```python
from build123d import *

# Parameters (mm, degrees)
F2_DEPTH  = 304.8
F4_D      = 14.2875
F4_DEPTH  = 6.35
F6_D      = 38.1
F6_DEPTH  = 6.35
F8_D      = 14.2875
F8_DEPTH  = 6.35
F10_D     = 31.75
F10_DEPTH = 6.35


with BuildPart() as f2:
    # F1 (on Right) → F2 (new body, symmetric)
    with BuildSketch(Plane.YZ):
        with BuildLine():
            Line((-177.776466, 50.8), (-266.676466, 50.8))
            ThreePointArc((-266.676466, 50.8), (-271.166595, 48.940128), (-273.026466, 44.45))
            Line((-273.026466, 44.45), (-273.026466, 37.770297))
            Line((-273.026466, 37.770297), (-273.026466, 6.35))
            ThreePointArc((-273.026466, 6.35), (-271.166595, 1.859872), (-266.676466, 0))
            Line((-266.676466, 0), (-177.776466, 0))
            ThreePointArc((-177.776466, 0), (-173.286338, 1.859872), (-171.426466, 6.35))
            Line((-171.426466, 6.35), (-171.426466, 44.45))
            ThreePointArc((-171.426466, 44.45), (-173.286338, 48.940128), (-177.776466, 50.8))
        make_face()
        with BuildLine():
            ThreePointArc((-266.671124, 38.101069), (-264.810874, 42.590506), (-260.321124, 44.45))
            Line((-260.321124, 44.45), (-182.185624, 44.45))
            ThreePointArc((-182.185624, 44.45), (-177.695496, 42.590128), (-175.835624, 38.1))
            Line((-175.835624, 38.1), (-175.835624, 12.7))
            ThreePointArc((-175.835624, 12.7), (-177.695496, 8.209872), (-182.185624, 6.35))
            Line((-182.185624, 6.35), (-260.325398, 6.35))
            ThreePointArc((-260.325398, 6.35), (-264.815904, 8.21025), (-266.675398, 12.701069))
            Line((-266.675398, 12.701069), (-266.671124, 38.101069))
        make_face(mode=Mode.SUBTRACT)
    extrude(amount=F2_DEPTH, both=True)

    # F4
    with Locations(Plane.XY.offset(50.8)):
        with Locations((-85.725, -222.226466), (85.725, -222.226466)):
            Hole(F4_D / 2, depth=F4_DEPTH)

    # F6
    with Locations(Plane.XY.offset(50.8)):
        with Locations((-228.6, -222.226466)):
            Hole(F6_D / 2, depth=F6_DEPTH)

    # F8
    with Locations(Plane(origin=(0, 0, 0), x_dir=(1, 0, 0), z_dir=(0, 0, -1))):
        with Locations((-228.6, 222.226466)):
            Hole(F8_D / 2, depth=F8_DEPTH)

    # F10
    with Locations(Plane(origin=(0, 0, 0), x_dir=(1, 0, 0), z_dir=(0, 0, -1))):
        with Locations((-85.725, 222.226466), (85.725, 222.226466)):
            Hole(F10_D / 2, depth=F10_DEPTH)


solid = f2.part
```
Input: part model. Units: mm. Frame: model coordinates. A direction names the side the tool comes from. Round coordinates to 2 decimals unless told otherwise and drop trailing zeros. Loops run counter-clockwise (first coordinate to the right, second up) from the corner with the lowest first, then second, coordinate; pieces in that order, holes last. Notation, with made-up numbers: (-28, 44.25) -> (-21, 44.25) arc R22 ccw to (-21, 66.25) -> close; hole circle Ø10 at (27.25, 48). An arc over 180 degrees is marked (long way). One line per item, written item: value.
(1) Section B-B (z = 19.5). Return the cut outline in (x, y), plus the area to 3 significant figures.
Geometry check:
outline: (-304.8, -273.03) -> (304.8, -273.03) -> (304.8, -266.67) -> (-304.8, -266.67) -> close; (-304.8, -175.84) -> (304.8, -175.84) -> (304.8, -171.43) -> (-304.8, -171.43) -> close
area: 6,560 mm2
(2) Material intervals for line 1 (Z direction, x = -90, y = -250.5); line 2 (Z direction, x = -235.5, y = -261); line 3 (Y direction, x = -256, z = 25.5), sorted ascending. Write a range as [from, to].
Geometry check:
line 1: [0, 6.35], [44.45, 50.8]
line 2: [0, 6.39], [44.41, 50.8]
line 3: [-273.03, -266.67], [-175.84, -171.43]
(3) Set-up query: faces 1 (the face through (-304.8, -226, 5)), 2 (the face through (4, -222, 44.45)), 3 (the face through (-214.56, -209.35, 47.58)), 4 (the face through (98.323, -212.567, 3.219)). Return all of +Z, -Z, +X, -X, +Y, -Y with unobstructed straight access to the full face (end or side cutting, diameter ignored); none if empty.
Geometry check:
face 1: +Z, -Z, -X, +Y, -Y
face 2: +X, -X
face 3: +Z
face 4: -Z
(4) Section D-D (x = 86). Return the cut outline in (y, z), plus the area to 3 significant figures.
Geometry check:
outline: (-273.03, 6.35) arc R6.35 ccw to (-266.68, 0) -> (-238.1, 0) -> (-238.1, 6.35) -> (-260.33, 6.35) arc R6.35 cw to (-266.68, 12.7) -> (-266.67, 38.1) arc R6.35 cw to (-260.32, 44.45) -> (-229.36, 44.45) -> (-229.36, 50.8) -> (-266.68, 50.8) arc R6.35 ccw to (-273.03, 44.45) -> close; (-215.09, 44.45) -> (-182.19, 44.45) arc R6.35 cw to (-175.84, 38.1) -> (-175.84, 12.7) arc R6.35 cw to (-182.19, 6.35) -> (-206.35, 6.35) -> (-206.35, 0) -> (-177.78, 0) arc R6.35 ccw to (-171.43, 6.35) -> (-171.43, 44.45) arc R6.35 ccw to (-177.78, 50.8) -> (-215.09, 50.8) -> close
area: 1,410 mm2
(5) Section C-C (x = 230). Return the cut outline in (y, z).
Geometry check:
outline: (-273.03, 6.35) arc R6.35 ccw to (-266.68, 0) -> (-177.78, 0) arc R6.35 ccw to (-171.43, 6.35) -> (-171.43, 44.45) arc R6.35 ccw to (-177.78, 50.8) -> (-266.68, 50.8) arc R6.35 ccw to (-273.03, 44.45) -> close; hole (-266.68, 12.7) arc R6.35 ccw to (-260.33, 6.35) -> (-182.19, 6.35) arc R6.35 ccw to (-175.84, 12.7) -> (-175.84, 38.1) arc R6.35 ccw to (-182.19, 44.45) -> (-260.32, 44.45) arc R6.35 ccw to (-266.67, 38.1) -> close
(6) Section A-A (x = -228.6). Return the cut outline in (y, z).
Geometry check:
outline: (-273.03, 6.35) arc R6.35 ccw to (-266.68, 0) -> (-229.37, 0) -> (-229.37, 6.35) -> (-260.33, 6.35) arc R6.35 cw to (-266.68, 12.7) -> (-266.67, 38.1) arc R6.35 cw to (-260.32, 44.45) -> (-241.28, 44.45) -> (-241.28, 50.8) -> (-266.68, 50.8) arc R6.35 ccw to (-273.03, 44.45) -> close; (-215.08, 0) -> (-177.78, 0) arc R6.35 ccw to (-171.43, 6.35) -> (-171.43, 44.45) arc R6.35 ccw to (-177.78, 50.8) -> (-203.18, 50.8) -> (-203.18, 44.45) -> (-182.19, 44.45) arc R6.35 cw to (-175.84, 38.1) -> (-175.84, 12.7) arc R6.35 cw to (-182.19, 6.35) -> (-215.08, 6.35) -> close
(7) Pin query (flat end, axial travel): pin 1 (11.5 mm diameter, centred on x = -228.6, y = -222.23, fed in from +Z) (3 decimals); pin 2 (18.5 mm diameter, centred on x = -85.72, y = -222.23, fed in from -Z). Return the tip coordinate at first contact, or that it passes through.
Geometry check:
pin 1: through
pin 2: z = 44.45
(8) Mould query, pull axis X, two halves, no side actions, for faces 5 (the face through (4, -222, 50.8)), 6 (the face through (304.8, -226, 5)), 7 (the face through (-89.021, -228.564, 47.581)). Classes: pulls with the +X half, pulls with the -X half, needs draft (parallel to the pull), parting line crosses it, or undercut.
Geometry check:
face 5: needs draft
face 6: pulls with the +X half
face 7: undercut
